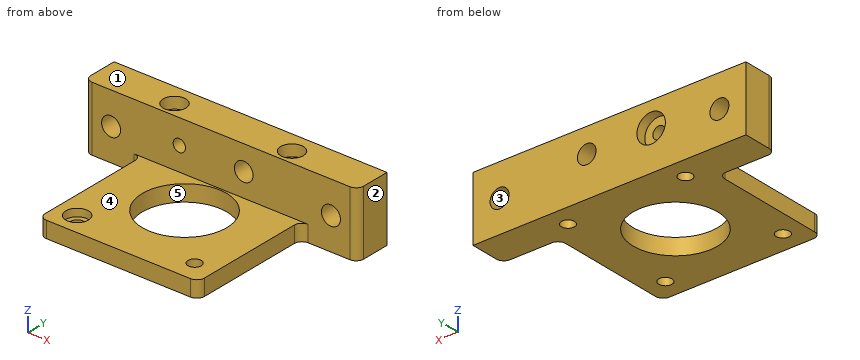
Autodesk Inventor part; units mm, degrees
ref_plane "Work Plane1" through (21, 0, 4.3) normal (1, 0, 0) x (0, 0, -1)
ref_plane "YZ Plane" through (0, 0, 0) normal (1, 0, 0) x (0, 1, 0)
ref_plane "XZ Plane" through (0, 0, 0) normal (0, 1, 0) x (-1, 0, 0)
sketch "Sketch1" plane through (0, 0, 0) normal (0, 0, 1) x (1, 0, 0)
  line L0 (0, 0) -> (42, 0)
  line L1 (42, 0) -> (42, 42)
  line L2 (42, 42) -> (0, 42)
  line L3 (0, 42) -> (0, 0)
  dimension "d0" = 42
  dimension "d1" = 42
extrude "Extrusion1" add sketch "Sketch1" along normal blind 4.3
sketch "Sketch2" plane through (0, 0, 4.3) normal (0, 0, 1) x (1, 0, 0)
  line L0 (0, 42) -> (0, 0)
  line L1 (42, 0) -> (42, 42)
  line L2 (0, 42) -> (42, 42)
  line L3 (42, 42) -> (42, 32.6)
  line L4 (42, 32.6) -> (0, 32.6)
  line L5 (0, 32.6) -> (0, 42)
  dimension "d4" = 9.4
extrude "Extrusion2" add sketch "Sketch2" along normal blind 12.7
sketch "Sketch3" plane through (0, 0, 4.3) normal (0, 0, 1) x (1, 0, 0)
  line L0 (0, 32.6) -> (0, 0)
  line L1 (0, 0) -> (42, 0)
  point P0 (21, 21)
  dimension "d7" = 21
  dimension "d8" = 21
hole "Hole1" at (21, 21, 4.3) direction (0, 0, -1) diameter 22.3 end through all
sketch "Sketch4" plane through (0, 0, 17) normal (0, 0, 1) x (1, 0, 0)
  line L0 (42, 42) -> (0, 42)
  line L1 (0, 42) -> (0, 32.6)
  line L2 (42, 32.6) -> (42, 42)
  line L3 (0, 0) -> (42, 0)
  point P0 (5.5, 36.5)
  point P1 (36.5, 36.5)
  dimension "d16" = 5.5
  dimension "d17" = 5.5
  dimension "d18" = 5.5
  dimension "d21" = 5.5
hole "Hole2" at (5.5, 36.5, 17) at (36.5, 36.5, 17) direction (0, 0, -1) diameter 3.5 end through all counterbore diameter 6 counterbore depth 3
sketch "Sketch5" plane through (0, 0, 4.3) normal (0, 0, 1) x (1, 0, 0)
  line L0 (0, 0) -> (42, 0)
  line L1 (0, 32.6) -> (0, 0)
  point P0 (5.5, 5.5)
  dimension "d31" = 5.5
  dimension "d32" = 5.5
hole "Hole3" at (5.5, 5.5, 4.3) direction (0, 0, -1) diameter 3.5 end through all counterbore diameter 6 counterbore depth 2
sketch "Sketch6" plane through (0, 0, 4.3) normal (0, 0, 1) x (1, 0, 0)
  line L0 (42, 0) -> (42, 32.6)
  line L1 (0, 0) -> (42, 0)
  point P0 (36.5, 5.5)
  dimension "d40" = 5.5
  dimension "d41" = 5.5
hole "Hole4" at (36.5, 5.5, 4.3) direction (0, 0, -1) diameter 3.5 end through all
sketch "Sketch7" plane through (0, 42, 0) normal (0, 1, 0) x (1, 0, 0)
  line L0 (0, -17) -> (42, -17)
  line L1 (42, 0) -> (42, -17)
  point P0 (0, 0)
  point P1 (27, -10.5)
  dimension "d49" = 6.5
  dimension "d50" = 15
hole "Hole5" at (27, 42, 10.5) direction (0, -1, 0) diameter 4.917 end through all
sketch "Sketch8" plane through (0, 42, 0) normal (0, 1, 0) x (1, 0, 0)
  line L0 (42, -17) -> (0, -17)
  line L1 (0, -4.3) -> (0, -17)
  point P0 (0, 0)
  point P1 (10, -10.5)
  dimension "d58" = 6.5
  dimension "d59" = 10
hole "Hole6" at (10, 42, 10.5) direction (0, -1, 0) diameter 3.242 end through all counterbore diameter 7.5 counterbore depth 2.5
sketch "Sketch9" plane through (42, 0, 0) normal (1, 0, 0) x (0, 0, -1)
  line L0 (-17, 32.6) -> (-17, 42)
  line L1 (0, 32.6) -> (-17, 32.6)
  line L2 (0, 42) -> (-17, 42)
  line L3 (0, 0) -> (0, 42)
extrude "Extrusion3" add sketch "Sketch9" along normal blind 15
sketch "Sketch10" plane through (0, 32.6, 4.3) normal (0, -1, 0) x (1, 0, 0)
  circle A0 centre (50, 4.2) radius 2.5
  line L0 (0, 12.7) -> (57, 12.7)
  line L1 (57, 12.7) -> (57, -4.3)
  point P0 (0, -4.3)
  dimension "d70" = 5
  dimension "d71" = 8.5
  dimension "d72" = 17
  dimension "d73" = 7
hole "Hole7" at (50, 32.6, 8.5) direction (0, 1, 0) diameter 5 end through all
ref_plane "Work Plane1" through (21, 0, 4.3) normal (1, 0, 0) x (0, 0, -1)
mirror "Mirror1" about plane through (21, 0, 4.3) normal (1, 0, 0) of "Hole7", "Extrusion3"
fillet "Fillet2" radius 2 6 edges at (-15, 32.6, 8.5) (0, 32.6, 2.15) (0, 0, 2.15) (42, 0, 2.15) (42, 32.6, 2.15) (57, 32.6, 8.5)
sketch "Sketch11" plane through (0, 0, 4.3) normal (0, 0, 1) x (1, 0, 0)
  line L0 (-6.1242, 27.6) -> (48.7334, 27.6)
  line L1 (55, 32.6) -> (-13, 32.6)
  line L2 (0, 27.6) -> (0, 2)
  arc A0 (0, 2) -> (2, 0) centre (2, 2) ccw
  line L3 (2, 0) -> (40, 0)
  arc A1 (40, 0) -> (42, 2) centre (40, 2) ccw
  line L4 (42, 2) -> (42, 27.6)
  point P0 (0, 0)
  dimension "d82" = 5
equation "\"d71\" = 0.5 * d72"
Source: CAD feature listing. Evaluate the final solid. Frame: model axes, mm. Face numbers are marked on the shaded views. A direction names the side the tool comes from. Round coordinates to 2 decimals unless told otherwise and drop trailing zeros. Order: outer loops, then holes, each group sorted by start corner. A loop starts at its lowest first (then second) coordinate and runs counter-clockwise, first axis right, second up. Notation, with made-up numbers: (42, 53.5) -> (66, 53.5) arc R12 ccw to (66, 68.5) -> close; hole circle Ø2 at (-8, 1). An arc over 180 degrees is marked (long way). Answer as CSV lines item,"result".
Item 1: Section A-A, the plane x = -8. Return loops of the section in (y, z), plus the area to 3 significant figures.
A:
outline,"(32.6, 0) -> (42, 0) -> (42, 6) -> (32.6, 6) -> close; (32.6, 11) -> (42, 11) -> (42, 17) -> (32.6, 17) -> close"
area,"113 mm²"
Item 2: Pull-direction query (X, two-part tool) for the marked faces 1, 2 and 3; classes: pulls with the +X half, pulls with the -X half, needs draft (parallel to the pull), parting line crosses it, or undercut.
A:
face 1,"needs draft"
face 2,"pulls with the +X half"
face 3,"undercut"
Item 3: Section B-B, the plane y = 21. Return loops of the section in (x, z), plus the area to 3 significant figures.
A:
outline,"(0, 0) -> (9.85, 0) -> (9.85, 4.3) -> (0, 4.3) -> close; (32.15, 0) -> (42, 0) -> (42, 4.3) -> (32.15, 4.3) -> close"
area,"84.7 mm²"
Item 4: Section C-C, the plane z = 5.25. Return loops of the section in (x, y).
A:
outline,"(-15, 34.6) arc R2 ccw to (-13, 32.6) -> (55, 32.6) arc R2 ccw to (57, 34.6) -> (57, 42) -> (-15, 42) -> close; hole circle Ø3.5 at (5.5, 36.5); hole circle Ø3.5 at (36.5, 36.5)"
Item 5: Section D-D, the plane y = 5.5. Return loops of the section in (x, z), plus the area to 4 significant figures.
A:
outline,"(0, 0) -> (3.75, 0) -> (3.75, 2.3) -> (2.5, 2.3) -> (2.5, 4.3) -> (0, 4.3) -> close; (7.25, 0) -> (34.75, 0) -> (34.75, 4.3) -> (8.5, 4.3) -> (8.5, 2.3) -> (7.25, 2.3) -> close; (38.25, 0) -> (42, 0) -> (42, 4.3) -> (38.25, 4.3) -> close"
area,"145.5 mm²"
Item 6: Reachability of the marked faces 4 and 5 from +Z, -Z, +X, -X, +Y, -Y: full face, straight path, thin tool, end or side. Return the list, or none.
A:
face 4,"+Z, +X, -X, -Y"
face 5,"+Z, -Z"
Item 7: Pin query (flat end, axial travel): pin 1 Ø8 at (x, z) = (-8, 8.5) entering from -Y; pin 2 Ø1.8 at (x, y) = (5.5, 37) entering from +Z; pin 3 Ø6 at (y, z) = (6, 4) entering from -X; pin 4 Ø4 at (x, z) = (10, 10.5) entering from +Y. Return the tip coordinate at first contact, or that it passes through.
A:
pin 1,"y = 32.6"
pin 2,"through"
pin 3,"x = 0"
pin 4,"y = 39.5"
Item 8: Line query: L1, parallel to X at y = 5.5, z = 1.55; L2, parallel to Z at x = 50, y = 37; L3, parallel to X at y = 41.15, z = 10.5. Output: solid intervals per line, ascending.
A:
L1,"0 to 3.75, 7.25 to 34.75, 38.25 to 42"
L2,"0 to 6, 11 to 17"
L3,"-15 to -9.5, -6.5 to 6.25, 13.75 to 24.54, 29.46 to 48.5, 51.5 to 57"
